```python
from build123d import *

# Parameters (mm, degrees)
F1_DEPTH  = 12.7
F4_DEPTH  = 3.81
F6_DEPTH  = 8.636
F8_DEPTH  = 25.4
F9_R      = 5.715
F10_DEPTH = 4.318


with BuildPart() as f1:
    # F0 (on Front) → F1 (new body)
    with BuildSketch(Plane.XZ):
        with BuildLine():
            Line((-11.43, -5.334), (11.43, -5.334))
            Line((11.43, -5.334), (11.43, 5.334))
            ThreePointArc((11.43, 5.334), (0, 16.764), (-11.43, 5.334))
            Line((-11.43, 5.334), (-11.43, -5.334))
        make_face()
    extrude(amount=F1_DEPTH)

    # F3 (on offset) → F4 (cut)
    with BuildSketch(Plane.XZ.offset(6.35)):
        with BuildLine():
            Line((-9.144, -5.334), (9.144, -5.334))
            Line((9.144, -5.334), (9.144, 5.334))
            ThreePointArc((9.144, 5.334), (0, 14.478), (-9.144, 5.334))
            Line((-9.144, 5.334), (-9.144, -5.334))
        make_face()
    extrude(amount=F4_DEPTH, mode=Mode.SUBTRACT)

    # F5 (on face) → F6 (cut)
    with BuildSketch(Plane.XZ.offset(12.7)):
        with BuildLine():
            Line((6.35, -5.334), (4.846011, 3.81))
            ThreePointArc((4.846011, 3.81), (0, 10.414), (-4.846011, 3.81))
            Line((-4.846011, 3.81), (-6.35, -5.334))
            Line((-6.35, -5.334), (6.35, -5.334))
        make_face()
    extrude(amount=-F6_DEPTH, mode=Mode.SUBTRACT)

    # F7 (on face) → F8 (cut)
    with BuildSketch(Plane.YZ.offset(11.43)):
        Polygon((-2.032, -2.286), (0, -3.302), (0, 14.732), (-2.032, 13.716), align=None)
    extrude(amount=-F8_DEPTH, mode=Mode.SUBTRACT)

    # F9 (on face) → F10 (cut, through all)
    with BuildSketch(Plane(origin=(0, -2.032, 0), x_dir=(-1, 0, 0), z_dir=(0, 1, 0))):
        with Locations((0, 5.334)):
            Circle(F9_R)
    extrude(amount=-F10_DEPTH, mode=Mode.SUBTRACT)


solid = f1.part
```
The model under review builds one solid part; all positions refer to its coordinate system, in mm. A direction names the side the tool comes from. Round coordinates to 2 decimals unless told otherwise and drop trailing zeros. Loops run counter-clockwise (first coordinate to the right, second up) from the corner with the lowest first, then second, coordinate; pieces in that order, holes last. Notation, with made-up numbers: M 34.5,0.5 L 88.5,0.5 A21 ccw 88.5,34.5 Z; hole C 72,-3 d10. An arc over 180 degrees is marked long. Put each result on its own line as item: value.
Q1. For pin 1 (11.5 mm diameter, centred on x = 0, z = 5.334, fed in from +Y); pin 2 (4 mm diameter, centred on x = 2.5, z = -1.5, fed in from -Y), all flat-tipped, find the tip position at first contact; note any pin that passes through.
Result set:
pin 1: stops at y = -2.03
pin 2: stops at y = -4.06
Q2. To check wall thickness, follow L1, parallel to X at y = -10, z = 1.75; L2, parallel to Y at x = 2.25, z = 11.5; L3, parallel to Z at x = 0, y = -3.8. State the ranges of each line that lie inside material, in increasing order.
Result set:
L1: x = -11.43 to -9.14, 9.14 to 11.43
L2: y = -12.7 to -10.16, -6.35 to -2.03
L3: z = -5.33 to -0.38, 11.05 to 16.76
Q3. Consider section A-A, the plane x = 0. Give the boundary of the cut face in (y, z).
Result set:
outline: M -12.7,10.41 L -10.16,10.41 L -10.16,14.48 L -6.35,14.48 L -6.35,11.05 L -2.03,11.05 L -2.03,13.72 L 0,14.73 L 0,16.76 L -12.7,16.76 Z; M -4.06,-5.33 L 0,-5.33 L 0,-3.3 L -2.03,-2.29 L -2.03,-0.38 L -4.06,-0.38 Z
Q4. Machinability: for faces 5 (the flat face through (5.704, -5.223, -1.404)), 6 (the flat face through (-0.1, -6.35, 11.3)), 7 (the cylindrical face through (-3.072, -4.161, 10.153)), 8 (the flat face through (0.2, -1, -2.8)), 9 (the cylindrical face through (0.25, -7.67, 16.76)), which of the approach directions +Z, -Z, +X, -X, +Y, -Y give a long, thin tool a straight path to every point of the face, cutting with its end or side? Answer none if there is none.
Result set:
face 5: -Z, -Y
face 6: -Z
face 7: +Y
face 8: +X, -X, +Y
face 9: +Z, +Y, -Y
Q5. Consider section B-B, the plane y = -7.25. Give the boundary of the cut face in (x, z).
Result set:
outline: M -11.43,-5.33 L -9.14,-5.33 L -9.14,5.33 A9.14 cw 9.14,5.33 L 9.14,-5.33 L 11.43,-5.33 L 11.43,5.33 A11.43 ccw -11.43,5.33 Z
Q6. Consider section C-C, the plane z = 1.25. Give the boundary of the cut face in (x, y).
Result set:
outline: M -11.43,-12.7 L -5.27,-12.7 L -5.27,-10.16 L -9.14,-10.16 L -9.14,-6.35 L -5.27,-6.35 L -5.27,-4.06 L -4,-4.06 L -4,-2.03 L -11.43,-2.03 Z; M 4,-4.06 L 5.27,-4.06 L 5.27,-6.35 L 9.14,-6.35 L 9.14,-10.16 L 5.27,-10.16 L 5.27,-12.7 L 11.43,-12.7 L 11.43,-2.03 L 4,-2.03 Z
Q7. Consider section D-D, the plane y = -11.75. Give the boundary of the cut face in (x, z), then the cut area to 3 significant figures.
Result set:
outline: M -11.43,-5.33 L -6.35,-5.33 L -4.85,3.81 A5.08 cw long 4.85,3.81 L 6.35,-5.33 L 11.43,-5.33 L 11.43,5.33 A11.43 ccw -11.43,5.33 Z
area: 291 mm²
Q8. Mouldability with a two-part tool opening along X and no side actions: class faces 1 (the flat face through (0.2, -2.032, 11.2)), 2 (the cylindrical face through (0.201, -8.228, 14.476)), 3 (the flat face through (-11.43, -8, 0)), 4 (the flat face through (-9.144, -8, 0)) as released by +X, released by -X, zero draft, split by the parting line, or undercut.
Result set:
face 1: zero draft
face 2: undercut
face 3: released by -X
face 4: undercut
